Autodesk Inventor part; units mm, degrees
ref_plane "YZ Plane" through (0, 0, 0) normal (1, 0, 0) x (0, 1, 0)
ref_plane "XZ Plane" through (0, 0, 0) normal (0, 1, 0) x (-1, 0, 0)
ref_plane "XY Plane" through (0, 0, 0) normal (0, 0, 1) x (1, 0, 0)
sketch "Sketch1" plane through (0, 0, 0) normal (0, 1, 0) x (-1, 0, 0)
  line L0 (0, 0) -> (61, 0)
  line L1 (61, 0) -> (61, -30)
  line L2 (61, -30) -> (0, -30)
  line L3 (0, -30) -> (0, 0)
  dimension "d0" = 30
  dimension "d1" = 61
extrude "Extrusion1" add sketch "Sketch1" along normal blind 13
sketch "Sketch4" plane through (0, 13, 0) normal (0, 1, 0) x (1, 0, 0)
  line L0 (-2, 2) -> (-59, 2)
  line L1 (-59, 2) -> (-59, 28)
  line L2 (-59, 28) -> (-2, 28)
  line L3 (-2, 28) -> (-2, 2)
  line L4 (-61, 0) -> (-61, 30)
  line L5 (0, 0) -> (-61, 0)
  line L6 (0, 30) -> (-61, 30)
  line L7 (0, 0) -> (0, 30)
  line L8 (-55, 24) -> (-59, 24)
  line L9 (-59, 24) -> (-59, 28)
  line L10 (-59, 28) -> (-55, 28)
  line L11 (-55, 28) -> (-55, 24)
  line L12 (-2, 28) -> (-6, 28)
  line L13 (-6, 28) -> (-6, 24)
  line L14 (-6, 24) -> (-2, 24)
  line L15 (-2, 24) -> (-2, 28)
  line L16 (-59, 6) -> (-55, 6)
  line L17 (-55, 6) -> (-55, 10)
  line L18 (-55, 10) -> (-59, 10)
  line L19 (-59, 10) -> (-59, 6)
  line L20 (-2, 6) -> (-6, 6)
  line L21 (-6, 6) -> (-6, 10)
  line L22 (-6, 10) -> (-2, 10)
  line L23 (-2, 10) -> (-2, 6)
  dimension "d18" = 2
  dimension "d19" = 2
  dimension "d20" = 2
  dimension "d21" = 2
  dimension "d26" = 4
  dimension "d27" = 4
  dimension "d30" = 4
  dimension "d31" = 4
  dimension "d53" = 4
  dimension "d54" = 4
  dimension "d57" = 0
  dimension "d61" = 6
  dimension "d139" = 4
  dimension "d140" = 4
  dimension "d141" = 0
  dimension "d142" = 6
extrude "Extrusion3" cut sketch "Sketch4" against normal blind 11 contours L0 L1 L16 L17 L18 L8 L11 L2 L13 L14 L3 L22 L21 L20
sketch "Sketch5" plane through (-61, 0, 0) normal (0, 0, 1) x (1, 0, 0)
  line L0 (16.5, 13) -> (27.5, 13)
  line L1 (27.5, 13) -> (27.5, 6)
  line L2 (27.5, 6) -> (16.5, 6)
  line L3 (16.5, 6) -> (16.5, 13)
  line L4 (61, 0) -> (61, 13)
  line L5 (59, 13) -> (2, 13)
  line L6 (0, 0) -> (0, 13)
  point P0 (55, 13)
  point P1 (6, 13)
  dimension "d38" = 11
  dimension "d39" = 7
  dimension "d41" = 0
  dimension "d48" = 16.5
extrude "Extrusion6" cut sketch "Sketch5" against normal through all
sketch "Sketch6" plane through (-61, 0, 0) normal (0, 0, 1) x (1, 0, 0)
  line L0 (55, 5) -> (59, 5)
  line L1 (59, 5) -> (59, 13)
  line L2 (59, 13) -> (55, 13)
  line L3 (55, 13) -> (55, 5)
  line L4 (61, 0) -> (61, 13)
  line L5 (27.5, 13) -> (61, 13)
  line L6 (61, 0) -> (0, 0)
  line L7 (2, 5) -> (6, 5)
  line L8 (6, 5) -> (6, 13)
  line L9 (6, 13) -> (2, 13)
  line L10 (2, 13) -> (2, 5)
  line L11 (0, 13) -> (16.5, 13)
  line L12 (0, 0) -> (0, 13)
  dimension "d45" = 6
  dimension "d47" = 0
  dimension "d50" = 4
  dimension "d63" = 5
  dimension "d64" = 0
  dimension "d65" = 4
  dimension "d66" = 5
  dimension "d67" = 6
extrude "Extrusion7" cut sketch "Sketch6" against normal blind 2
sketch "Sketch9" plane through (0, 2, 0) normal (0, 1, 0) x (1, 0, 0)
  line L0 (-55, 2) -> (-55, 0)
  line L1 (-55, 0) -> (-44.5, 0)
  line L2 (-44.5, 0) -> (-44.5, 2)
  line L3 (-44.5, 2) -> (-55, 2)
  line L4 (-6, 0) -> (-6, 2)
  line L5 (-6, 2) -> (-33.5, 2)
  line L6 (-33.5, 2) -> (-33.5, 0)
  line L7 (-33.5, 0) -> (-6, 0)
  line L8 (-44.5, 2) -> (-55, 2)
  line L9 (-50.5, 4) -> (-46.5, 4)
  line L10 (-46.5, 4) -> (-46.5, 8)
  line L11 (-46.5, 8) -> (-50.5, 8)
  line L12 (-50.5, 8) -> (-50.5, 4)
  line L13 (-46.5, 22) -> (-46.5, 26)
  line L14 (-46.5, 26) -> (-50.5, 26)
  line L15 (-50.5, 26) -> (-50.5, 22)
  line L16 (-50.5, 22) -> (-46.5, 22)
  line L17 (-27.5, 4) -> (-27.5, 8)
  line L18 (-27.5, 8) -> (-31.5, 8)
  line L19 (-31.5, 8) -> (-31.5, 4)
  line L20 (-31.5, 4) -> (-27.5, 4)
  line L21 (-27.5, 22) -> (-27.5, 26)
  line L22 (-27.5, 26) -> (-31.5, 26)
  line L23 (-31.5, 26) -> (-31.5, 22)
  line L24 (-31.5, 22) -> (-27.5, 22)
  line L25 (-55, 28) -> (-6, 28)
  line L26 (-44.5, 30) -> (-61, 30)
  dimension "d202" = 4
  dimension "d203" = 4
  dimension "d204" = 2
  dimension "d205" = 2
  dimension "d208" = 18
  dimension "d211" = 19
  dimension "d231" = 2
  dimension "d232" = 30
  dimension "d233" = 2
extrude "Extrusion8" add sketch "Sketch9" along normal blind 2.4 contours L12 L11 L10 L9 | L16 L15 L14 L13 | L20 L19 L18 L17 | L24 L23 L22 L21
chamfer "Chamfer2" distance 1 angle 45 2 edges at (-55, 9, 0) (-6, 9, 0)
fillet "Fillet1" radius 1 34 edges at (-61, 6.5, 0) (0, 6.5, 0) (0, 6.5, -30) (-61, 6.5, -30) (-55, 7.5, -24) (-59, 7.5, -24) (-55, 7.5, -28) (-59, 7.5, -6) (-55, 7.5, -6) (-55, 7.5, -10) (-59, 7.5, -10) (-2, 7.5, -6) (-6, 7.5, -6) (-6, 7.5, -10) (-2, 7.5, -10) (-6, 7.5, -24) (-2, 7.5, -24) (-6, 7.5, -28) (-31.5, 3.2, -22) (-27.5, 3.2, -22) (-46.5, 3.2, -22) (-50.5, 3.2, -22) (-46.5, 3.2, -8) (-50.5, 3.2, -8) (-31.5, 3.2, -8) (-27.5, 3.2, -8) (-46.5, 3.2, -4) (-50.5, 3.2, -4) (-31.5, 3.2, -4) (-27.5, 3.2, -4) (-50.5, 3.2, -26) (-46.5, 3.2, -26) (-31.5, 3.2, -26) (-27.5, 3.2, -26)
sketch "Sketch7" plane through (0, 13, 0) normal (0, 1, 0) x (1, 0, 0)
  circle A0 centre (-57, 26) radius 0.75
  circle A1 centre (-4, 26) radius 0.75
  circle A2 centre (-57, 8) radius 0.75
  line L0 (-55, 24) -> (-55, 28)
  line L1 (-59, 24) -> (-55, 24)
  line L2 (-6, 24) -> (-2, 24)
  line L3 (-6, 28) -> (-6, 24)
  line L4 (-55, 6) -> (-55, 10)
  line L5 (-59, 6) -> (-55, 6)
  circle A3 centre (-4, 8) radius 0.75
  line L6 (-6, 10) -> (-6, 6)
  line L7 (-6, 6) -> (-2, 6)
  point P0 (0, 0)
  dimension "d68" = 1.5
  dimension "d70" = 1.5
  dimension "d71" = 1.5
  dimension "d72" = 2
  dimension "d73" = 2
  dimension "d74" = 2
  dimension "d75" = 2
  dimension "d78" = 2
  dimension "d79" = 2
  dimension "d143" = 1.5
  dimension "d145" = 2
  dimension "d146" = 2
hole "Hole1" at (-57, 13, -26) at (-4, 13, -26) at (-57, 13, -8) at (-4, 13, -8) direction (0, -1, 0) diameter 1.7 depth 10
sketch "Sketch14" plane through (0, 4.4, 0) normal (0, 1, 0) x (1, 0, 0)
  line L0 (-50.5, 7) -> (-50.5, 5)
  line L1 (-47.5, 8) -> (-49.5, 8)
  point P0 (0, 0)
  point P1 (-48.5, 6)
  point P2 (-49, 3)
  point P3 (-48.5, 24)
  point P4 (-29.5, 6)
  point P5 (-29.5, 24)
  point P6 (-49, 4)
  dimension "d214" = 2
  dimension "d215" = 2
  dimension "d218" = 18
  dimension "d221" = 19
hole "Hole4" at (-48.5, 4.4, -6) at (-48.5, 4.4, -24) at (-29.5, 4.4, -6) at (-29.5, 4.4, -24) direction (0, -1, 0) diameter 1.7 depth 2 tip angle 118
properties part number "Link Adapter"
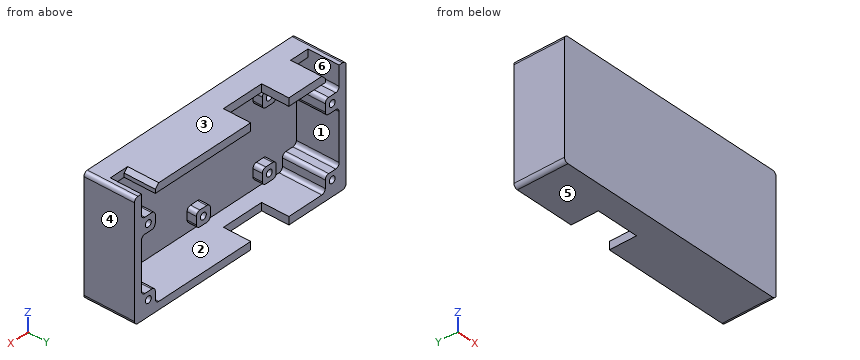
Here's how the part is built. I have some questions about the finished solid (model axes, mm). Face numbers are marked on the shaded views. A direction names the side the tool comes from. Round coordinates to 2 decimals unless told otherwise and drop trailing zeros. Loops run counter-clockwise (first coordinate to the right, second up) from the corner with the lowest first, then second, coordinate; pieces in that order, holes last.
1. Suppose I cut it at C-C, the plane x = -40.5. Please give me the cut outline in (y, z), and give its area (3 significant figures).
Answers:
outline: (0, -30) - (6, -30) - (6, -28) - (2, -28) - (2, -2) - (6, -2) - (6, 0) - (0, 0) - close
area: 76.0 mm2
2. Will these pins go through, and if not, where does the flat tip stop? pin 1 (1.5 mm diameter, centred on x = -57, z = -8, fed in from -Y); pin 2 (4.5 mm diameter, centred on x = -30.5, z = -5.5, fed in from +Y); pin 3 (0.6 mm diameter, centred on x = -56.5, y = 7.5, fed in from +Z).
Answers:
pin 1: stops at y = 0
pin 2: stops at y = 4.4
pin 3: stops at z = -6
3. Suppose I cut it at A-A, the plane z = -14.25. Please give me the cut outline in (x, y), and give its area (3 significant figures).
Answers:
outline: (-61, 0) - (0, 0) - (0, 13) - (-2, 13) - (-2, 2) - (-59, 2) - (-59, 13) - (-61, 13) - close
area: 166 mm2
4. Suppose I cut it at B-B, the plane y = 10.25. Give the number of separate pieces and of enclosed holes in the cut face, and give its area (3 significant figures).
Answers:
separate pieces: 4
enclosed holes: 4
area: 341 mm2
5. For the marked faces 5 and 6, which set-ups out of +Z, -Z, +X, -X, +Y, -Y let a thin tool reach every point of the face, with its end or its side?
Answers:
face 5: -Z, +X, -X, +Y, -Y
face 6: +Y
6. Thinking about a two-plate mould opening in Z: for the marked faces 1, 2, 3 and 4, which applies, released by +Z, released by -Z, zero draft, split by the parting line, or undercut?
Answers:
face 1: undercut
face 2: undercut
face 3: released by +Z
face 4: zero draft
7. Suppose I cut it at D-D, the plane x = -4. Please give me the cut outline in (y, z), and give its area (3 significant figures).
Answers:
outline: (0, -30) - (13, -30) - (13, -26.85) - (3, -26.85) - (3, -25.15) - (13, -25.15) - (13, -24) - (2, -24) - (2, -10) - (13, -10) - (13, -8.85) - (3, -8.85) - (3, -7.15) - (13, -7.15) - (13, -6) - (2, -6) - (2, -2) - (5, -2) - (5, 0) - (0, 0) - close
area: 142 mm2
8. If I drill on probe 1 along Z at (x, y) = (-57, 11); probe 2 along X at (y, z) = (9, -26); probe 3 along Z at (x, y) = (-48.5, 3.6), over which ranges is the centre line in solid material (lowest first)?
Answers:
probe 1: z = -30 to -26.85, -25.15 to -24, -10 to -8.85, -7.15 to -6
probe 2: x = -61 to -57.85, -56.15 to -55, -6 to -4.85, -3.15 to 0
probe 3: z = -30 to -28, -26 to -24.85, -23.15 to -22, -8 to -6.85, -5.15 to -4, -2 to 0
